Input: part model. Units: mm. Frame: model coordinates. Coordinates: 2 decimals unless noted, no trailing zeros. Loops run counter-clockwise (first coordinate to the right, second up) from the corner with the lowest first, then second, coordinate; pieces in that order, holes last. Notation, with made-up numbers: (81, -11) - (123, -11) arc R9 ccw to (123, -4) - close; hole circle Ø10 at (89.25, -25.5). An arc over 180 degrees is marked (long way). Use one line per item in the form item = value.
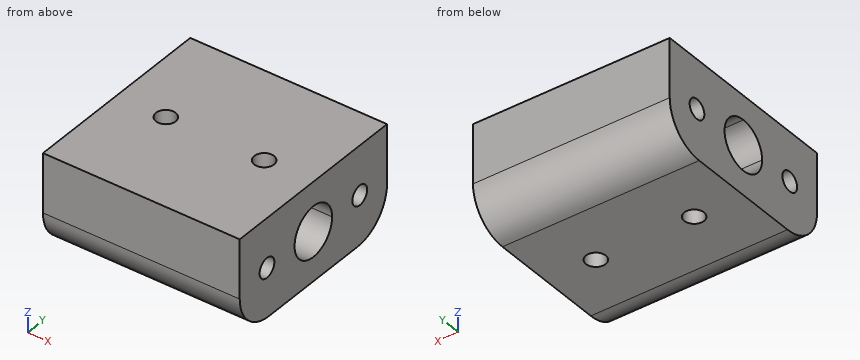
from build123d import *

# Parameters (mm, degrees)
F0_R     = 1.27
F1_DEPTH = 12.7
F2_DEPTH = 6.35
F3_DEPTH = 6.35
F4_R     = 1.27
F5_DEPTH = 50.8
F6_R     = 5.08


with BuildPart() as f1:
    # F0 (on Top) → F1 (new body)
    with BuildSketch(Plane.XY):
        Polygon((-12.7, 0), (0, 0), (0, 12.7), (-25.4, 12.7), (-25.4, 0), align=None)
        with Locations((-19.05, 6.35)):
            Circle(F0_R, mode=Mode.SUBTRACT)
        with BuildLine():
            ThreePointArc((-5.08, 6.35), (-6.35, 5.08), (-7.62, 6.35))
            ThreePointArc((-7.62, 6.35), (-6.35, 7.62), (-5.08, 6.35))
        make_face(mode=Mode.SUBTRACT)
    extrude(amount=F1_DEPTH)

    # F2 (add): a face of the model
    f2_faces = [f1.faces().sort_by_distance(p)[0] for p in [
        (-12.7, 0, 6.35),
    ]]
    extrude(f2_faces, amount=F2_DEPTH)

    # F3 (add): a face of the model
    f3_faces = [f1.faces().sort_by_distance(p)[0] for p in [
        (-12.7, 12.7, 6.35),
    ]]
    extrude(f3_faces, amount=F3_DEPTH)

    # F4 (on face) → F5 (cut)
    with BuildSketch(Plane.YZ):
        with Locations((-1.651, 6.35)):
            Circle(F4_R)
        with BuildLine():
            Line((6.35, 6.35), (6.35, 9.5885))
            ThreePointArc((6.35, 9.5885), (4.0600346891, 8.6399653109), (3.1115, 6.35))
            Line((3.1115, 6.35), (6.35, 6.35))
        make_face()
        with BuildLine():
            ThreePointArc((9.5885, 6.35), (8.6399653109, 8.6399653109), (6.35, 9.5885))
            Line((6.35, 9.5885), (6.35, 6.35))
            Line((6.35, 6.35), (9.5885, 6.35))
        make_face()
        with BuildLine():
            Line((9.5885, 6.35), (6.35, 6.35))
            Line((6.35, 6.35), (3.1115, 6.35))
            ThreePointArc((3.1115, 6.35), (6.35, 3.1115), (9.5885, 6.35))
        make_face()
        with BuildLine():
            ThreePointArc((15.621, 6.35), (14.351, 7.62), (13.081, 6.35))
            ThreePointArc((13.081, 6.35), (14.351, 5.08), (15.621, 6.35))
        make_face()
    extrude(amount=-F5_DEPTH, mode=Mode.SUBTRACT)

    # F6
    f6_edges = [f1.edges().sort_by_distance(p)[0] for p in [
        (-12.7, -6.35, 0),
        (-12.7, 19.05, 0),
    ]]
    fillet(f6_edges, radius=F6_R)


solid = f1.part
Q1. First-contact query: P1, Ø1.5, axis at y = 4.5, z = 6, coming from the +X side. Flat tip, straight axial feed; report the tip coordinate or a pass-through.
Check values:
P1 = through
Q2. Cut plane B-B, the plane z = 6. Return loops of the section in (x, y).
Check values:
outline = (-25.4, -6.35) - (0, -6.35) - (0, -2.87) - (-25.4, -2.87) - close; (-25.4, -0.43) - (0, -0.43) - (0, 3.13) - (-25.4, 3.13) - close; (-25.4, 9.57) - (0, 9.57) - (0, 13.13) - (-25.4, 13.13) - close; (-25.4, 15.57) - (0, 15.57) - (0, 19.05) - (-25.4, 19.05) - close
Q3. Ray query, line 1 along X through (y, z) = (6.35, 11.05); line 2 along Y through (x, z) = (-14.5, 7.5); line 3 along Z through (x, y) = (-11.5, 14.25). Return the intervals inside material, ascending. Write a range as [from, to].
Check values:
line_1 = [-25.4, -20.32], [-17.78, -7.62], [-5.08, 0]
line_2 = [-6.35, -2.19], [-1.11, 3.32], [9.38, 13.81], [14.89, 19.05]
line_3 = [0.01, 5.08], [7.62, 12.7]
Q4. Cut plane C-C, the plane x = -21.75. Return loops of the section in (y, z).
Check values:
outline = (-6.35, 5.08) arc R5.08 ccw to (-1.27, 0) - (13.97, 0) arc R5.08 ccw to (19.05, 5.08) - (19.05, 12.7) - (-6.35, 12.7) - close; hole circle Ø2.54 at (-1.65, 6.35); hole circle Ø6.48 at (6.35, 6.35); hole circle Ø2.54 at (14.35, 6.35)
Q5. Cut plane A-A, the plane x = -6.35. Return loops of the section in (y, z), then the cut area to 3 significant figures.
Check values:
outline = (-6.35, 5.08) arc R5.08 ccw to (-1.27, 0) - (5.08, 0) - (5.08, 3.37) arc R3.24 cw to (5.08, 9.33) - (5.08, 12.7) - (-6.35, 12.7) - close; (7.62, 0) - (13.97, 0) arc R5.08 ccw to (19.05, 5.08) - (19.05, 12.7) - (7.62, 12.7) - (7.62, 9.33) arc R3.24 cw to (7.62, 3.37) - close; hole circle Ø2.54 at (-1.65, 6.35); hole circle Ø2.54 at (14.35, 6.35)
area = 252 mm²
Q6. Cut plane D-D, the plane z = 10.25. Return loops of the section in (x, y).
Check values:
outline = (-25.4, -6.35) - (0, -6.35) - (0, 19.05) - (-25.4, 19.05) - close; hole circle Ø2.54 at (-19.05, 6.35); hole circle Ø2.54 at (-6.35, 6.35)
